```python
from build123d import *

# Parameters (mm, degrees)
F0_R     = 8
F1_DEPTH = 150
F2_R     = 6
F3_DEPTH = 150.001
F4_SIZE  = 0.2
F5_SIZE  = 0.2


with BuildPart() as f1:
    # F0 (on Right) → F1 (new body)
    with BuildSketch(Plane.YZ):
        Circle(F0_R)
    extrude(amount=F1_DEPTH)

    # F2 (on face) → F3 (cut, through all)
    with BuildSketch(Plane.YZ.offset(150)):
        Circle(F2_R)
    extrude(amount=-F3_DEPTH, mode=Mode.SUBTRACT)

    # F4
    f4_edges = [f1.edges().sort_by_distance(p)[0] for p in [
        (150, -8, 0),
    ]]
    chamfer(f4_edges, length=F4_SIZE)

    # F5
    f5_edges = [f1.edges().sort_by_distance(p)[0] for p in [
        (0, -8, 0),
    ]]
    chamfer(f5_edges, length=F5_SIZE)


solid = f1.part
```
Geometry: final body of the model. Coordinates: model frame, mm. Coordinates: 2 decimals unless noted, no trailing zeros. Order: outer loops, then holes, each group sorted by start corner. A loop starts at its lowest first (then second) coordinate and runs counter-clockwise, first axis right, second up.
Item 1: Draft query along Z for faces 1 (the face through (0, 4, -5)), 2 (the face through (76, -6, 0)), 3 (the face through (73.95, -1.73, -7.81)). Return one class per face: released by +Z, released by -Z, zero draft, split by the parting line, or undercut.
Answer:
face 1: zero draft
face 2: undercut
face 3: split by the parting line
Item 2: Contact query for flat-ended pins moving along their axis: P1, Ø6, axis at x = 77, y = 5, coming from the +Z side; P2, Ø2, axis at x = 24.5, z = 6, coming from the -Y side (3 decimals). Output: stop coordinate, or through.
Answer:
P1: stops at z = 7.75
P2: stops at y = -6.245
Item 3: Material intervals for line 1 along Y through (x, z) = (82, -0.5); line 2 along Z through (x, y) = (115.5, 0); line 3 along Z through (x, y) = (99, -3.25), sorted ascending.
Answer:
line 1: y = -7.98 to -5.98, 5.98 to 7.98
line 2: z = -8 to -6, 6 to 8
line 3: z = -7.31 to -5.04, 5.04 to 7.31
Item 4: Section query C-C (x = 98.5). Output: boundary loops of the cut face in (y, z).
Answer:
outline: circle Ø16 at (0, 0); hole circle Ø12 at (0, 0)
Item 5: Section query A-A (z = 0). Output: boundary loops of the cut face in (x, y), then the cut area to 3 significant figures.
Answer:
outline: (0, -7.8) - (0.2, -8) - (149.8, -8) - (150, -7.8) - (150, -6) - (0, -6) - close; (0, 6) - (150, 6) - (150, 7.8) - (149.8, 8) - (0.2, 8) - (0, 7.8) - close
area: 600 mm2
